Geometry check sheet. Reference: the model listing, model coordinates, mm. Face numbers are marked on the shaded views. A direction names the side the tool comes from. Coordinates: 2 decimals unless noted, no trailing zeros. Order: outer loops, then holes, each group sorted by start corner. A loop starts at its lowest first (then second) coordinate and runs counter-clockwise, first axis right, second up. Notation, with made-up numbers: M 38.25,-25.5 L 63.25,-25.5 A19 cw 63.25,4.5 Z; hole C 5.25,-13.75 d9. An arc over 180 degrees is marked long. Use CSV: the item, a comma, the result in double quotes. Start each with the question number.
```python
from build123d import *

# Parameters (mm, degrees)
F0_W      = 25.908
F0_H      = 78.74
F1_DEPTH  = 11.43
F3_DEPTH  = 13.97
F6_W      = 12.954
F6_H      = 16.51
F7_DEPTH  = 11.43
F11_DEPTH = 2.54


with BuildPart() as f1:
    # F0 (on Top) → F1 (new body)
    with BuildSketch(Plane.XY):
        Rectangle(F0_W, F0_H)
    extrude(amount=-F1_DEPTH)

    # F2 (on Top) → F3 (join)
    with BuildSketch(Plane.XY):
        Polygon((15.494, 41.91), (-15.494, 41.91), (-15.494, -39.37), (-12.954, -39.37), (-12.954, 39.37), (12.954, 39.37), (12.954, -39.37), (15.494, -39.37), align=None)
    extrude(amount=-F3_DEPTH)

    # F4 (on face) → F5 (revolve, cut)
    with BuildSketch(Plane(origin=(0, 0, -11.43), x_dir=(1, 0, 0), z_dir=(0, 0, -1))):
        Polygon((3.429, -39.37), (5.08, 39.37), (0, 39.37), (0, -39.37), align=None)
    revolve(axis=Axis((0, 0, -11.43), (0, -1, 0)), mode=Mode.SUBTRACT)

    # F6 (on Top) → F7 (join)
    with BuildSketch(Plane.XY):
        with Locations((6.477, -47.625)):
            Rectangle(F6_W, F6_H)
        with Locations((-6.477, -47.625)):
            Rectangle(F6_W, F6_H)
    extrude(amount=-F7_DEPTH)

    # F8 (on face) → F9 (revolve, cut)
    with BuildSketch(Plane(origin=(0, 0, -11.43), x_dir=(1, 0, 0), z_dir=(0, 0, -1))):
        with BuildLine():
            Line((6.35, 55.88), (0, 55.88))
            Line((0, 55.88), (0, 39.37))
            Line((0, 39.37), (5.08, 39.37))
            Line((5.08, 39.37), (6.35, 39.37))
            ThreePointArc((6.35, 39.37), (9.0440768363, 40.4859231637), (10.16, 43.18))
            Line((10.16, 43.18), (10.16, 52.07))
            ThreePointArc((10.16, 52.07), (9.0440768363, 54.7640768363), (6.35, 55.88))
        make_face()
    revolve(axis=Axis((0, -47.625, -11.43), (0, -1, 0)), mode=Mode.SUBTRACT)

    # F10 (on face) → F11 (join)
    with BuildSketch(Plane.XZ.offset(55.88)):
        with BuildLine():
            Line((12.954, 0), (-12.954, 0))
            Line((-12.954, 0), (-12.954, -11.43))
            Line((-12.954, -11.43), (-6.35, -11.43))
            ThreePointArc((-6.35, -11.43), (0, -5.08), (6.35, -11.43))
            Line((6.35, -11.43), (12.954, -11.43))
            Line((12.954, -11.43), (12.954, 0))
        make_face()
        with BuildLine():
            ThreePointArc((6.35, -11.43), (0, -5.08), (-6.35, -11.43))
            Line((-6.35, -11.43), (-3.81, -11.43))
            ThreePointArc((-3.81, -11.43), (0, -7.62), (3.81, -11.43))
            Line((3.81, -11.43), (6.35, -11.43))
        make_face()
    extrude(amount=F11_DEPTH)


solid = f1.part
```
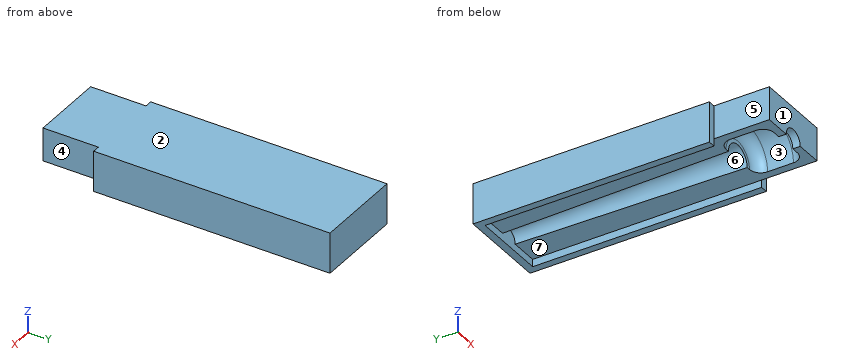
1) Material ranges on line 1 along Y through (x, z) = (-2, -6); line 2 along X through (y, z) = (9, -11.75); line 3 along Z through (x, y) = (-5.5, 25), recorded low to high.
2) Section check B-B on x = 0. Record the boundary of the cut face in (y, z).
3) Section check C-C on y = -5.5. Record the boundary of the cut face in (x, z).
4) Section check D-D on y = -21.5. Record the boundary of the cut face in (x, z).
5) Set-up check for the marked faces 4, 5, 6 and 7: record each of +Z, -Z, +X, -X, +Y, -Y from which the full face is reachable in a straight line by a thin tool's end or side.
6) Draft check along Y on the marked faces 1, 2 and 3. Enter one of: +Y half, -Y half, draft (parallel to the pull), parting line (faces both ways), or undercut.
7) Section check A-A on z = -12.5. Record the boundary of the cut face in (x, y).
8) Gauge pin test, flat ends, axial feed: P1, Ø1.3, axis at x = 14, z = -7, coming from the -Y side; P2, Ø5, axis at x = 9.5, y = -10.5, coming from the -Z side. Record the tip position at first contact, or that the pin passes through.
Results are:
1,line 1,"y = -58.42 to -55.88, -39.37 to 41.91"
1,line 2,"x = -15.49 to -12.95, 12.95 to 15.49"
1,line 3,"z = -11.43 to 0"
2,outline,"M -58.42,-7.62 L -55.88,-7.62 L -55.88,-5.08 A3.81 cw -52.07,-1.27 L -43.18,-1.27 A3.81 cw -39.37,-5.08 L -39.37,-6.35 L 39.37,-8 L 39.37,-13.97 L 41.91,-13.97 L 41.91,0 L -58.42,0 Z"
3,outline,"M -15.49,-13.97 L -12.95,-13.97 L -12.95,-11.43 L -4.37,-11.43 A4.37 cw 4.37,-11.43 L 12.95,-11.43 L 12.95,-13.97 L 15.49,-13.97 L 15.49,0 L -15.49,0 Z"
4,outline,"M -15.49,-13.97 L -12.95,-13.97 L -12.95,-11.43 L -4.71,-11.43 A4.71 cw 4.71,-11.43 L 12.95,-11.43 L 12.95,-13.97 L 15.49,-13.97 L 15.49,0 L -15.49,0 Z"
5,face 4,"+Z, -Z, +X, -Y"
5,face 5,"+Z, -Z, -X, -Y"
5,face 6,"-Z"
5,face 7,"-Z, -Y"
6,face 1,"-Y half"
6,face 2,"draft"
6,face 3,"undercut"
7,outline,"M -15.49,-39.37 L -12.95,-39.37 L -12.95,39.37 L 12.95,39.37 L 12.95,-39.37 L 15.49,-39.37 L 15.49,41.91 L -15.49,41.91 Z"
8,P1,"stops at y = -39.37"
8,P2,"stops at z = -11.43"
